Input: dimensioned drawing with shaded views. Units: mm. Origin: part minimum x, y, z. A direction names the side the tool comes from. Coordinates: 2 decimals unless noted, no trailing zeros. Order: outer loops, then holes, each group sorted by start corner. A loop starts at its lowest first (then second) coordinate and runs counter-clockwise, first axis right, second up. Notation, with made-up numbers: (18.5, -29) - (77.5, -29) arc R36 ccw to (77.5, 10) - close; hole circle Ø1 at (43, 68). An arc over 180 degrees is marked (long way). One line per question, with ' | ' between items. Start each with the question number.
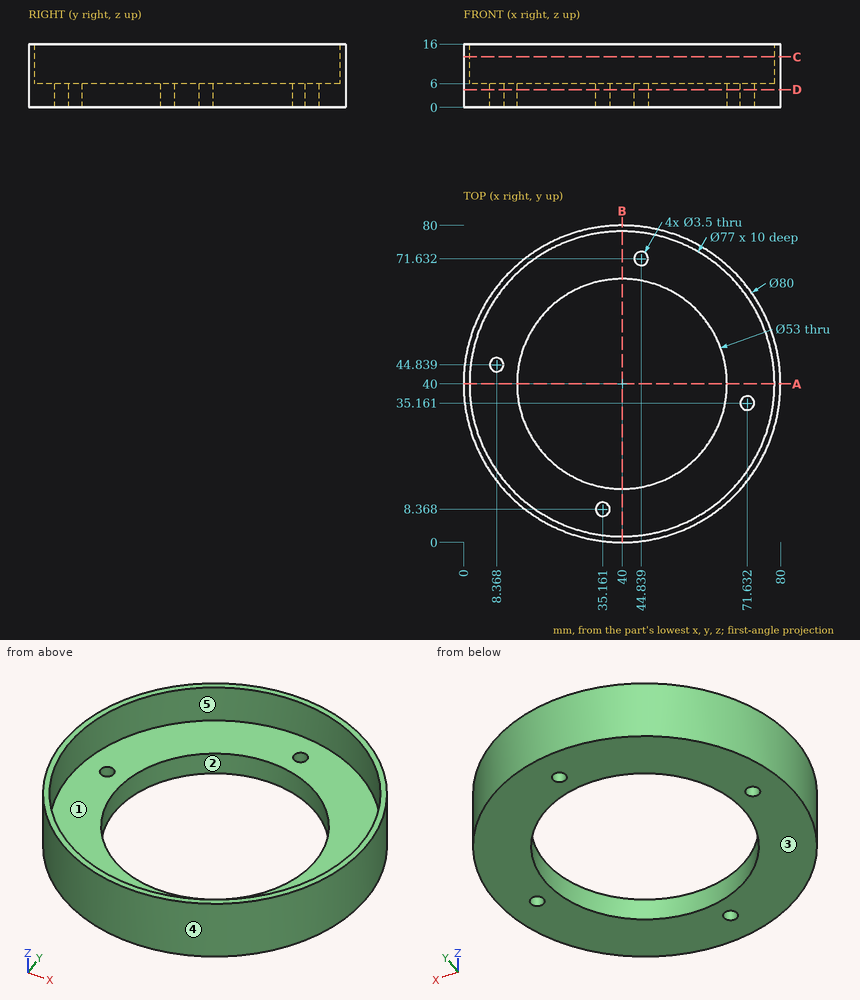
(1) Material intervals for line 1 along Y through (x, z) = (40, 2.9); line 2 along Y through (x, z) = (40, 13.75); line 3 along Z through (x, y) = (53.5, 12.5), sorted ascending. Write a range as from..to.
(2) Section D-D (z = 4.5). Output: boundary loops of the cut face in (x, y).
(3) Draft query along Y for the marked faces 3, 4 and 5. Return one class per face: +Y half, -Y half, draft (parallel to the pull), parting line (faces both ways), or undercut.
(4) Section C-C (z = 12.75). Output: boundary loops of the cut face in (x, y).
(5) Pin query (flat end, axial travel): pin 1 (3 mm diameter, centred on x = 35.16, y = 8.37, fed in from +Z); pin 2 (1.5 mm diameter, centred on x = 28, z = 10.5, fed in from +Y) (1 decimal); pin 3 (3 mm diameter, centred on x = 48.5, z = 8.5, fed in from +Y); pin 4 (8 mm diameter, centred on x = 59.5, z = 14.5, fed in from +Y) (1 decimal). Return the tip coordinate at first contact, or that it passes through.
(6) Reachability of the marked faces 1 and 2 from +Z, -Z, +X, -X, +Y, -Y: full face, straight path, thin tool, end or side. Return the list, or none.
(7) Section A-A (y = 40). Output: boundary loops of the cut face in (x, z), then the cut area to 3 significant figures.
Worked answers:
1) line 1: y = 0..13.5, 66.5..80 | line 2: y = 0..1.5, 78.5..80 | line 3: z = 0..6
2) outline: circle Ø80 at (40, 40); hole circle Ø3.5 at (8.37, 44.84); hole circle Ø53 at (40, 40); hole circle Ø3.5 at (35.16, 8.37); hole circle Ø3.5 at (44.84, 71.63); hole circle Ø3.5 at (71.63, 35.16)
3) face 3: draft | face 4: parting line | face 5: undercut
4) outline: circle Ø80 at (40, 40); hole circle Ø77 at (40, 40)
5) pin 1: passes through | pin 2: stops at y = 78.4 | pin 3: stops at y = 79.38 | pin 4: stops at y = 76.9
6) face 1: +Z | face 2: +Z, -Z
7) outline: (0, 0) - (13.5, 0) - (13.5, 6) - (1.5, 6) - (1.5, 16) - (0, 16) - close; (66.5, 0) - (80, 0) - (80, 16) - (78.5, 16) - (78.5, 6) - (66.5, 6) - close | area: 192 mm²
